Check sheet for the modelled part. Datum: model origin and axes. Units: mm. Coordinates: 2 decimals unless noted, no trailing zeros. Order: outer loops, then holes, each group sorted by start corner. A loop starts at its lowest first (then second) coordinate and runs counter-clockwise, first axis right, second up.
from build123d import *

# Parameters (mm, degrees)
SKETCH1_R           = 17.5
SKETCH1_R_2         = 12.5
BOSS_EXTRUDE1_DEPTH = 280
SKETCH8_R           = 17.5
BOSS_EXTRUDE3_DEPTH = 10
SKETCH9_R           = 12.55
CUT_EXTRUDE2_DEPTH  = 899.5


with BuildPart() as part:
    # Sketch1 → Boss-Extrude1 (new, symmetric)
    with BuildSketch(Plane(origin=(0, 0, 0), x_dir=(1, 0, 0), z_dir=(0, 1, 0))):
        with Locations(Location((0, 0, 0), (0, 0, 270))):
            Circle(SKETCH1_R)
        with Locations(Location((0, 0, 0), (0, 0, 270))):
            Circle(SKETCH1_R_2, mode=Mode.SUBTRACT)
    extrude(amount=BOSS_EXTRUDE1_DEPTH, both=True)

    # Sketch8 → Boss-Extrude3 (add)
    with BuildSketch(Plane.XZ.offset(280)):
        with Locations(Location((0, 0, 0), (0, 0, 270))):
            Circle(SKETCH8_R)
    extrude(amount=BOSS_EXTRUDE3_DEPTH)

    # Sketch9 → Cut-Extrude2 (cut)
    with BuildSketch(Plane(origin=(-32.302786122, 416.289190775, -45.221901395), x_dir=(-0.9768887275019512, 0, 0.2137484832217963), z_dir=(0, 1, 0))):
        with Locations(Location((-21.890114798, 51.081437247, 0), (0, 0, 77.657886074))):
            Circle(SKETCH9_R)
    extrude(amount=-CUT_EXTRUDE2_DEPTH, mode=Mode.SUBTRACT)


solid = part.part
(1) Cross-section at A-A (z = 0). Enter the section's corners in (x, y).
Filled in:
outline: (-17.5, -290) - (-12.55, -290) - (-12.55, 280) - (-17.5, 280) - close; (12.55, -290) - (17.5, -290) - (17.5, 280) - (12.55, 280) - close
(2) Cross-section at C-C (y = -208). Enter the section's corners in (x, z).
Filled in:
outline: circle Ø35 at (0, 0); hole circle Ø25.1 at (0, 0)
(3) Thickness scan on probe 1 along X at (y, z) = (49, 0); probe 2 along Z at (x, y) = (0.5, -260.5); probe 3 along X at (y, z) = (-12, -1.5). Record the ranges inside material, lowest first.
Filled in:
probe 1: x = -17.5 to -12.55, 12.55 to 17.5
probe 2: z = -17.49 to -12.54, 12.54 to 17.49
probe 3: x = -17.44 to -12.46, 12.46 to 17.44
(4) Release check for a two-part mould opening along Z. For faces 1 (the cylindrical face through (-7.636, -1.01, -9.959)), 2 (the flat face through (-11, 280, 8)) record: +Z half, -Z half, draft (parallel to the pull), parting line (faces both ways), or undercut.
Filled in:
face 1: undercut
face 2: draft
(5) Go/stop test with flat-tipped pins: P1, Ø8, axis at y = -158, z = -12, coming from the -X side; P2, Ø8, axis at x = 5, y = -60.5, coming from the -Z side; P3, Ø12, axis at x = 10.5, y = -41.5, coming from the -Z side; P4, Ø12, axis at y = -133.5, z = -1.5, coming from the -X side. Record where each tip stops, or that it passes through.
Filled in:
P1: stops at x = -15.56
P2: stops at z = -17.47
P3: stops at z = -16.91
P4: stops at x = -17.5
(6) Cross-section at B-B (x = 0). Enter the section's corners in (y, z).
Filled in:
outline: (-290, -17.5) - (280, -17.5) - (280, -12.55) - (-290, -12.55) - close; (-290, 12.55) - (280, 12.55) - (280, 17.5) - (-290, 17.5) - close
